Here's how the part is built. I have some questions about the finished solid (model axes, mm). Round coordinates to 2 decimals unless told otherwise and drop trailing zeros. Loops run counter-clockwise (first coordinate to the right, second up) from the corner with the lowest first, then second, coordinate; pieces in that order, holes last. Notation, with made-up numbers: M -36.5,-32 L 12.5,-32 A22 ccw 12.5,-4 Z; hole C -17.5,88 d1. An arc over 180 degrees is marked long. Use a Markdown table: item, result.
from build123d import *

# Parameters (mm, degrees)
SKETCH_2_W          = 150
SKETCH_2_H          = 150
CUT_EXTRUDE_1_DEPTH = 70
SHELL_1_T           = -4
SKETCH_3_R          = 80
SKETCH_3_R_2        = 66
EXTRUDE_1_DEPTH     = 4


with BuildPart() as part:
    # 草图1 → 旋转1 (revolve)
    with BuildSketch(Plane.XY):
        with BuildLine():
            Line((0, 70), (0, -70))
            ThreePointArc((0, -70), (70, 0), (0, 70))
        make_face()
    revolve(axis=Axis((0, 70, 0), (0, -1, 0)))

    # 草图2 → 切除-拉伸1 (cut)
    with BuildSketch(Plane(origin=(0, 0, 0), x_dir=(1, 0, 0), z_dir=(0, 1, 0))):
        Rectangle(SKETCH_2_W, SKETCH_2_H)
    extrude(amount=CUT_EXTRUDE_1_DEPTH, mode=Mode.SUBTRACT)

    # 抽壳1
    shell_1_openings = [part.faces().sort_by_distance(p)[0] for p in [
        (0, 0, 0),
    ]]
    offset(amount=SHELL_1_T, openings=shell_1_openings, kind=Kind.INTERSECTION)

    # 草图3 → 凸台-拉伸1 (add)
    with BuildSketch(Plane(origin=(0, 0, 0), x_dir=(1, 0, 0), z_dir=(0, 1, 0))):
        with Locations(Location((0, 0, 0), (0, 0, 270))):
            Circle(SKETCH_3_R)
        Circle(SKETCH_3_R_2, mode=Mode.SUBTRACT)
    extrude(amount=-EXTRUDE_1_DEPTH)


solid = part.part
1. We'd pull the mould along Z, two halves only. Please class faces 1 (the face through (66, 0, 11)), 2 (the face through (-78.1, -1.97, -17.34)): +Z half, -Z half, draft (parallel to the pull), parting line (faces both ways), or undercut.
Answer sheet:
| item | result |
|---|---|
| face 1 | draft |
| face 2 | parting line |
2. For pin 1 Ø12 at (y, z) = (-43.5, -21) entering from +X; pin 2 Ø4 at (y, z) = (-28.5, 4.5) entering from -X; pin 3 Ø2 at (x, z) = (24.5, 29.5) entering from +Y, each with a flat end and sliding along its axis, tell me the tip position at first contact or that it passes through.
Answer sheet:
| item | result |
|---|---|
| pin 1 | x = 55.77 |
| pin 2 | x = -64.64 |
| pin 3 | y = -52.99 |
3. I need wall thicknesses on probe 1 along Y at (x, z) = (-28, -69.5); probe 2 along Z at (x, y) = (-40.5, -20); probe 3 along Z at (x, y) = (17, -32). Which ranges of each line are inside material? Lowest first, please. Write a range as from..to.
Answer sheet:
| item | result |
|---|---|
| probe 1 | -4..0 |
| probe 2 | -53.48..-48.12, 48.12..53.48 |
| probe 3 | -59.89..-55.16, 55.16..59.89 |
4. Imagine slicing it at C-C, the plane y = -17.5. Write out the boundary of the cut face in (x, z).
Answer sheet:
| item | result |
|---|---|
| outline | C 0,0 d135.55; hole C 0,0 d127.28 |
